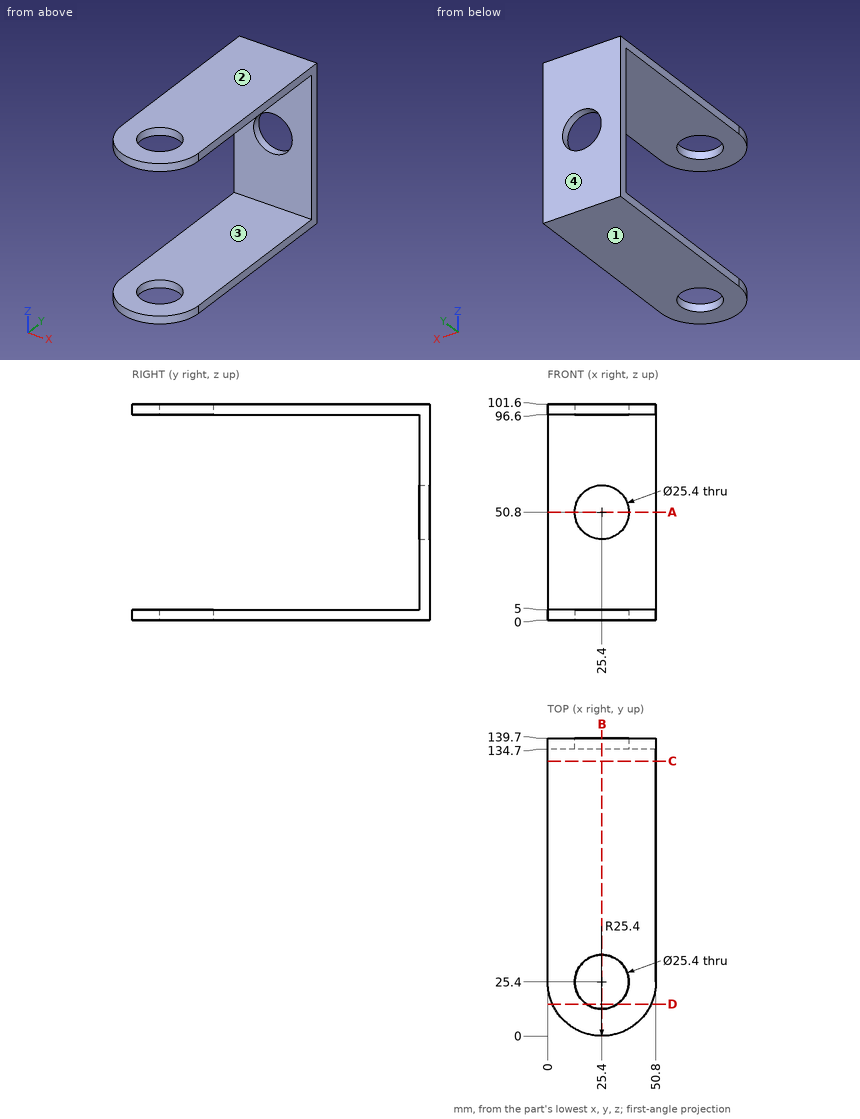
Answer from the drawing. Dimensions are ordinates in mm from the lowest x, y and z of the part. Round coordinates to 2 decimals unless told otherwise and drop trailing zeros. Loops run counter-clockwise (first coordinate to the right, second up) from the corner with the lowest first, then second, coordinate; pieces in that order, holes last. Notation, with made-up numbers: (29.5, 5.25) - (39.5, 5.25) arc R25 cw to (39.5, 29.25) - close; hole circle Ø3 at (17.5, 33.5). An arc over 180 degrees is marked (long way). Return JSON: item names as keys, results as strings. Group by question number.
1. The part is cut by section D-D on y = 15. Determine the outline of the cut face in (x, z).
2. This flat-tipped pin is pushed along its axis until it touches: P1, Ø1, axis at x = 9, z = 30, coming from the -Y side. Where does it stop, or does it pass through?
3. The mould has two halves that part along Z. Classify the marked faces 1, 2, 3 and 4: pulls with the +Z half, pulls with the -Z half, needs draft (parallel to the pull), parting line crosses it, or undercut.
4. The part is cut by section C-C on y = 129. Determine the outline of the cut face in (x, z), then the cut area to 3 significant figures.
5. The part is cut by section B-B on x = 25.4. Determine the outline of the cut face in (y, z), then the cut area to 3 significant figures.
6. Consider probe 1 along Z at (x, y) = (4.5, 50); probe 2 along Y at (x, z) = (25, 100); probe 3 along X at (y, z) = (25.4, 98.35). Determine where each line is inside the solid, lowest interval first.
7. The part is cut by section A-A on z = 50.8. Determine the outline of the cut face in (x, y).
Resolved:
{
 "1": {"outline": "(2.23, 0) - (18.11, 0) - (18.11, 5) - (2.23, 5) - close; (2.23, 96.6) - (18.11, 96.6) - (18.11, 101.6) - (2.23, 101.6) - close; (32.69, 0) - (48.57, 0) - (48.57, 5) - (32.69, 5) - close; (32.69, 96.6) - (48.57, 96.6) - (48.57, 101.6) - (32.69, 101.6) - close"},
 "2": {"P1": "stops at y = 134.7"},
 "3": {"face 1": "pulls with the -Z half", "face 2": "pulls with the +Z half", "face 3": "undercut", "face 4": "needs draft"},
 "4": {"outline": "(0, 0) - (50.8, 0) - (50.8, 5) - (0, 5) - close; (0, 96.6) - (50.8, 96.6) - (50.8, 101.6) - (0, 101.6) - close", "area": "508 mm²"},
 "5": {"outline": "(0, 0) - (12.7, 0) - (12.7, 5) - (0, 5) - close; (0, 96.6) - (12.7, 96.6) - (12.7, 101.6) - (0, 101.6) - close; (38.1, 0) - (139.7, 0) - (139.7, 38.1) - (134.7, 38.1) - (134.7, 5) - (38.1, 5) - close; (38.1, 96.6) - (134.7, 96.6) - (134.7, 63.5) - (139.7, 63.5) - (139.7, 101.6) - (38.1, 101.6) - close", "area": "1,470 mm²"},
 "6": {"probe 1": "z = 0 to 5, 96.6 to 101.6", "probe 2": "y = 0 to 12.71, 38.09 to 139.7", "probe 3": "x = 0 to 12.7, 38.1 to 50.8"},
 "7": {"outline": "(0, 134.7) - (12.7, 134.7) - (12.7, 139.7) - (0, 139.7) - close; (38.1, 134.7) - (50.8, 134.7) - (50.8, 139.7) - (38.1, 139.7) - close"}
}
